Read the model definition and answer for the solid it produces. Units are mm, in the model's axes. Coordinates: 2 decimals unless noted, no trailing zeros. Write each loop counter-clockwise with the first axis right and the second up, starting at its lowest first coordinate (ties: lowest second). Pieces come first, ordered by that corner, then holes. Notation, with made-up numbers: (0.25, -28) -> (43.25, -28) arc R10 cw to (43.25, -19) -> close; hole circle Ø11 at (-34.5, 78.25). An arc over 180 degrees is marked (long way). Use CSV: the item, a comma, the result in double quotes. Start each with the question number.
from build123d import *

# Parameters (mm, degrees)
ESQUISSE1_R        = 7
ESQUISSE1_R_2      = 3.5
BOSS_EXTRU_1_DEPTH = 1
CONG_1_R           = 0.2
CONG_2_R           = 0.2


with BuildPart() as part:
    # Esquisse1 → Boss.-Extru.1 (new body)
    with BuildSketch(Plane.XY):
        Circle(ESQUISSE1_R)
        Circle(ESQUISSE1_R_2, mode=Mode.SUBTRACT)
    extrude(amount=BOSS_EXTRU_1_DEPTH)

    # Congé1
    cong_1_edges = [part.edges().sort_by_distance(p)[0] for p in [
        (-7, 0, 0),
        (-7, 0, 1),
        (-3.5, 0, 1),
    ]]
    fillet(cong_1_edges, radius=CONG_1_R)

    # Congé2
    cong_2_edges = [part.edges().sort_by_distance(p)[0] for p in [
        (-3.5, 0, 0),
    ]]
    fillet(cong_2_edges, radius=CONG_2_R)


solid = part.part
1) Section C-C, the plane z = 0.6 is taken. Give the vertices of the cut face in (x, y).
2) Find the intervals of material crossed by line 1 along Y through (x, z) = (0, 0.4); line 2 along Y through (x, z) = (-1.25, 0.8); line 3 along X through (y, z) = (-0.25, 0.6), in increasing order.
3) The mould has two halves that part along X. Classify faces 1 (the face through (6.466, -2.681, 0.496)), 2 (the face through (3, -3, 1)), 3 (the face through (3.233, -1.341, 0.496)): pulls with the +X half, pulls with the -X half, needs draft (parallel to the pull), parting line crosses it, or undercut.
4) This flat-tipped pin is pushed along its axis until it touches: pin 1 (4 mm diameter, centred on x = 0, y = 0, fed in from -Z). Where does it stop, or does it pass through?
5) Section A-A, the plane y = 0 is taken. Give the vertices of the cut face in (x, z).
The answers:
1,outline,"circle Ø14 at (0, 0); hole circle Ø7 at (0, 0)"
2,line 1,"y = -7 to -3.5, 3.5 to 7"
2,line 2,"y = -6.89 to -3.27, 3.27 to 6.89"
2,line 3,"x = -7 to -3.49, 3.49 to 7"
3,face 1,"parting line crosses it"
3,face 2,"needs draft"
3,face 3,"undercut"
4,pin 1,"passes through"
5,outline,"(-7, 0.2) arc R0.2 ccw to (-6.8, 0) -> (-3.7, 0) arc R0.2 ccw to (-3.5, 0.2) -> (-3.5, 0.8) arc R0.2 ccw to (-3.7, 1) -> (-6.8, 1) arc R0.2 ccw to (-7, 0.8) -> close; (3.5, 0.2) arc R0.2 ccw to (3.7, 0) -> (6.8, 0) arc R0.2 ccw to (7, 0.2) -> (7, 0.8) arc R0.2 ccw to (6.8, 1) -> (3.7, 1) arc R0.2 ccw to (3.5, 0.8) -> close"
